Geometry: see drawing. Coordinates: mm, zero at the bounding-box minimum. A direction names the side the tool comes from. Coordinates: 2 decimals unless noted, no trailing zeros. Write each loop counter-clockwise with the first axis right and the second up, starting at its lowest first coordinate (ties: lowest second). Pieces come first, ordered by that corner, then holes. Notation, with made-up numbers: M 11.25,-11 L 24.25,-11 A34 cw 24.25,26 Z; hole C -22,32 d3. An arc over 180 degrees is marked long. Answer as CSV lines item,"result". Start each with the question number.
1. Section B-B on z = 30. Return the cut outline in (x, y).
2. Section D-D on x = 32.5. Return the cut outline in (y, z) (3 decimals), plus the area to 3 significant figures.
3. Reachability of the marked faces 5, 6 and 7 from +Z, -Z, +X, -X, +Y, -Y: full face, straight path, thin tool, end or side. Return the list, or none.
4. Line query: probe 1 along Z at (x, y) = (100, 27); probe 2 along Y at (x, z) = (12.5, 12); probe 3 along X at (y, z) = (29.75, 20). Output: solid intervals per line, ascending. Write a range as [from, to].
5. Section A-A on x = 15. Return the cut outline in (y, z), plus the area to 3 significant figures.
6. Contact query for flat-ended pins moving along their axis: pin 1 Ø20 at (x, z) = (107, 18.5) entering from +Y; pin 2 Ø12 at (x, z) = (102.5, 21.5) entering from -Y; pin 3 Ø1 at (x, y) = (57.5, 8.5) entering from -Z; pin 4 Ø2 at (y, z) = (21, 35) entering from -X. Output: stop coordinate, or through.
7. Mould query, pull axis Y, two halves, no side actions, for the marked faces 1, 2, 3 and 4. Classes: pulls with the +Y half, pulls with the -Y half, needs draft (parallel to the pull), parting line crosses it, or undercut.
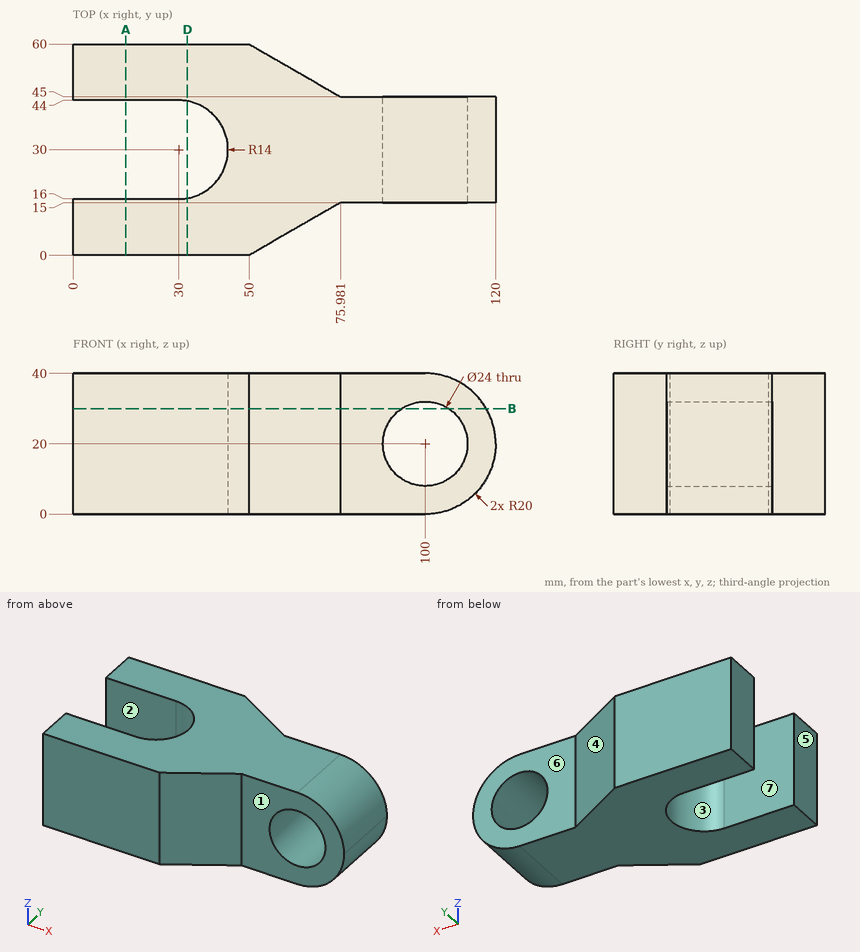
Values:
1,outline,"M 0,0 L 50,0 L 75.98,15 L 93.37,15 L 93.37,45 L 75.98,45 L 50,60 L 0,60 L 0,44 L 30,44 A14 cw 30,16 L 0,16 Z; M 106.63,15 L 117.32,15 L 117.32,45 L 106.63,45 Z"
2,outline,"M 0,0 L 16.225,0 L 16.225,40 L 0,40 Z; M 43.775,0 L 60,0 L 60,40 L 43.775,40 Z"
2,area,"1,300 mm²"
3,face 5,"+Z, -Z, -X, +Y, -Y"
3,face 6,"+Z, -Z, +X, +Y"
3,face 7,"+Z, -Z, -X"
4,probe 1,"[0, 8], [32, 40]"
4,probe 2,"[0, 16], [44, 60]"
4,probe 3,"[44, 88], [112, 120]"
5,outline,"M 0,0 L 16,0 L 16,40 L 0,40 Z; M 44,0 L 60,0 L 60,40 L 44,40 Z"
5,area,"1,280 mm²"
6,pin 1,"y = 45"
6,pin 2,"through"
6,pin 3,"z = 0"
6,pin 4,"x = 39.8"
7,face 1,"pulls with the -Y half"
7,face 2,"undercut"
7,face 3,"undercut"
7,face 4,"pulls with the +Y half"
